```python
from build123d import *

# Parameters (mm, degrees)
SKETCH1_W                       = 150
SKETCH1_H                       = 40
BOSS_EXTRUDE1_DEPTH             = 2
SKETCH2_W                       = 150
SKETCH2_H                       = 40
BOSS_EXTRUDE2_DEPTH             = 2
CUT_EXTRUDE1_DEPTH              = 12.7
CUT_EXTRUDE1_DEPTH_BACK         = 2.3
BOSS_EXTRUDE3_DEPTH             = 9
BOSS_EXTRUDE4_REACH             = 32.803
BOSS_EXTRUDE4_DIRECTION_2_REACH = 11.197
CUT_EXTRUDE2_DEPTH              = 9
CUT_EXTRUDE3_DEPTH              = 2
SKETCH8_W                       = 10.5
SKETCH8_H                       = 9.597099162
SKETCH8_H_2                     = 6.297094949
BOSS_EXTRUDE5_DEPTH             = 9


with BuildPart() as part:
    # Sketch1 → Boss-Extrude1 (new body)
    with BuildSketch(Plane.XY):
        with Locations((53.542293618, 10.802935989)):
            Rectangle(SKETCH1_W, SKETCH1_H)
        with BuildLine():
            Line((107.411442145, 19.39470724), (107.411442145, 16.563139449))
            ThreePointArc((107.411442145, 16.563139449), (99.879507012, 8.827431039), (90.278173099, 3.889251358))
            ThreePointArc((90.278173099, 3.889251358), (87.976829975, 4.107947017), (85.862026946, 5.041550847))
            Line((85.862026946, 5.041550847), (83.564794922, 4.425052911))
            Line((83.564794922, 4.425052911), (81.157246557, 3.778949869))
            ThreePointArc((81.157246557, 3.778949869), (80.265596131, 1.871389792), (78.431111832, 0.8377103))
            Line((78.431111832, 0.8377103), (63.171073337, -3.257558326))
            ThreePointArc((63.171073337, -3.257558326), (60.782240037, -2.264409978), (59.531114294, 0))
            Line((59.531114294, 0), (51.260116039, 0))
            ThreePointArc((51.260116039, 0), (50.153419477, -2.317171365), (47.784117276, -3.307356952))
            Line((47.784117276, -3.307356952), (15.784117324, -3.309106743))
            ThreePointArc((15.784117324, -3.309106743), (13.343545232, -2.355539788), (12.195889194, 0))
            Line((12.195889194, 0), (0, 0))
            Line((0, 0), (0, 7.1))
            Line((0, 7.1), (11.639427583, 7.1))
            ThreePointArc((11.639427583, 7.1), (13.95708374, 11.772480363), (17.201849985, 15.85599537))
            ThreePointArc((17.201849985, 15.85599537), (17.97614749, 16.386455083), (18.8959739, 16.573119247))
            Line((18.8959739, 16.573119247), (44.695973562, 16.568946787))
            ThreePointArc((44.695973562, 16.568946787), (45.539742509, 16.358143902), (46.249834575, 15.85599537))
            ThreePointArc((46.249834575, 15.85599537), (49.049011998, 12.449181276), (51.19972816, 8.6))
            Line((51.19972816, 8.6), (59.697013712, 8.6))
            ThreePointArc((59.697013712, 8.6), (60.947722352, 11.657213146), (63.162897087, 14.107483583))
            ThreePointArc((63.162897087, 14.107483583), (63.865840812, 15.804539858), (65.562897087, 16.507483583))
            Line((65.562897087, 16.507483583), (72.962892379, 16.499136125))
            ThreePointArc((72.962892379, 16.499136125), (74.529247661, 15.732293003), (75.162897087, 14.107483583))
            ThreePointArc((75.162897087, 14.107483583), (76.943795958, 13.247586891), (78.431584017, 11.944701709))
            Line((78.431584017, 11.944701709), (84.544097467, 13.585089744))
            ThreePointArc((84.544097467, 13.585089744), (85.264438336, 15.182566708), (86.505516367, 16.419720272))
            ThreePointArc((86.505516367, 16.419720272), (94.138787289, 25.104262189), (104.023703334, 19.106218503))
            Line((104.023703334, 19.106218503), (107.411442145, 19.39470724))
        make_face(mode=Mode.SUBTRACT)
    extrude(amount=BOSS_EXTRUDE1_DEPTH)

    # Sketch2 → Boss-Extrude2 (add)
    with BuildSketch(Plane.XY):
        with Locations((53.542293618, 10.802935989)):
            Rectangle(SKETCH2_W, SKETCH2_H)
    extrude(amount=-BOSS_EXTRUDE2_DEPTH)

    # Sketch3 → Cut-Extrude1 (cut, two sides)
    with BuildSketch(Plane(origin=(0, 0, 0), x_dir=(1, 0, 0), z_dir=(0, 1, 0))) as cut_extrude1_sk:
        with BuildLine():
            Line((0, -0.8), (0, -17.6))
            ThreePointArc((0, -17.6), (-15.540418318, -9.2), (0, -0.8))
        make_face()
    extrude(amount=CUT_EXTRUDE1_DEPTH, mode=Mode.SUBTRACT)
    extrude(cut_extrude1_sk.sketch, amount=-CUT_EXTRUDE1_DEPTH_BACK, mode=Mode.SUBTRACT)

    # Sketch4 → Boss-Extrude3 (add)
    with BuildSketch(Plane.XY):
        Polygon((0, 7.1), (0, 12.7), (-12.497856815, 12.7), (-15.345436436, 12.7), (-15.345436436, 16.697099162), (-12.345546973, 16.697099162), (4, 16.697099162), (11, 16.697099162), (11, 7.1), align=None)
        Polygon((0, 0), (0, -2.3), (-12.497856815, -2.3), (-15.345436436, -2.3), (-15.345436436, -6.297094949), (-12.345436436, -6.297094949), (4, -6.297094949), (11, -6.297094949), (11, 0), align=None)
    extrude(amount=BOSS_EXTRUDE3_DEPTH)

    # Boss-Extrude4: up to this face of the body (flat: up to its plane)
    boss_extrude4_end = Plane(part.part.faces().sort_by_distance((-2.172718218, 16.697099162, 5.5))[0])
    # Sketch5 → Boss-Extrude4 (add, up to the picked face)
    with BuildSketch(Plane(origin=(0, 0, 0), x_dir=(1, 0, 0), z_dir=(0, 1, 0)), mode=Mode.PRIVATE) as boss_extrude4_sk1:
        with BuildLine():
            Line((-15.290812019, -9), (-19.400060853, -9))
            Line((-19.400060853, -9), (-19.400060853, -2))
            Line((-19.400060853, -2), (-12.345436436, -2))
            ThreePointArc((-12.345436436, -2), (-14.524477307, -5.20278927), (-15.290812019, -9))
        make_face()
    boss_extrude4_tool1 = split(extrude(boss_extrude4_sk1.sketch, amount=BOSS_EXTRUDE4_REACH, mode=Mode.PRIVATE), bisect_by=boss_extrude4_end, keep=Keep.BOTH, mode=Mode.PRIVATE)
    add(boss_extrude4_tool1.solids().sort_by_distance((-16.816054, 0, 5.171228))[0])

    # Boss-Extrude4 direction 2: up to this face of the body (flat: up to its plane)
    boss_extrude4_direction_2_end = Plane(part.part.faces().sort_by_distance((-2.172718218, -6.297094949, 5.5))[0])
    # Sketch5 → Boss-Extrude4 direction 2 (add, up to the picked face)
    with BuildSketch(Plane(origin=(0, 0, 0), x_dir=(1, 0, 0), z_dir=(0, 1, 0)), mode=Mode.PRIVATE) as boss_extrude4_direction_2_sk1:
        with BuildLine():
            Line((-15.290812019, -9), (-19.400060853, -9))
            Line((-19.400060853, -9), (-19.400060853, -2))
            Line((-19.400060853, -2), (-12.345436436, -2))
            ThreePointArc((-12.345436436, -2), (-14.524477307, -5.20278927), (-15.290812019, -9))
        make_face()
    boss_extrude4_direction_2_tool1 = split(extrude(boss_extrude4_direction_2_sk1.sketch, amount=-BOSS_EXTRUDE4_DIRECTION_2_REACH, mode=Mode.PRIVATE), bisect_by=boss_extrude4_direction_2_end, keep=Keep.BOTH, mode=Mode.PRIVATE)
    add(boss_extrude4_direction_2_tool1.solids().sort_by_distance((-16.816054, 0, 5.171228))[0])

    # Sketch6 → Cut-Extrude2 (cut)
    with BuildSketch(Plane.XY.offset(9)):
        Polygon((0, 7.1), (0, 12.7), (-15.290812019, 12.7), (-15.290812019, 13.2), (0.5, 13.2), (0.5, 7.1), align=None)
        Polygon((-15.290812019, -2.3), (0, -2.3), (0, 0), (0.5, 0), (0.5, -2.8), (-15.290812019, -2.8), align=None)
    extrude(amount=-CUT_EXTRUDE2_DEPTH, mode=Mode.SUBTRACT)

    # Sketch7 → Cut-Extrude3 (cut)
    with BuildSketch(Plane.XY.offset(2)):
        Polygon((11.639427583, 7.1), (11.639427583, 26.1), (109.411442143, 26.1), (109.411442143, -4.30823185), (11.639427583, -4.30823185), align=None)
    extrude(amount=-CUT_EXTRUDE3_DEPTH, mode=Mode.SUBTRACT)

    # Sketch8 → Boss-Extrude5 (add)
    with BuildSketch(Plane.XY.offset(9)):
        with Locations((5.75, 11.898549581)):
            Rectangle(SKETCH8_W, SKETCH8_H)
        with Locations((5.75, -3.148547475)):
            Rectangle(SKETCH8_W, SKETCH8_H_2)
    extrude(amount=BOSS_EXTRUDE5_DEPTH)


solid = part.part
```
Work out the finished part from the listing and answer in its coordinate system (mm). A direction names the side the tool comes from. Round coordinates to 2 decimals unless told otherwise and drop trailing zeros. Order: outer loops, then holes, each group sorted by start corner. A loop starts at its lowest first (then second) coordinate and runs counter-clockwise, first axis right, second up.
Q1. A cutting plane is placed at C-C, the plane x = 67.5. Determine the outline of the cut face in (y, z).
Solution:
outline: (-9.2, -2) - (30.8, -2) - (30.8, 2) - (26.1, 2) - (26.1, 0) - (-4.31, 0) - (-4.31, 2) - (-9.2, 2) - close
Q2. A cutting plane is placed at B-B, the plane y = 2.5. Determine the outline of the cut face in (x, z), then the cut area to 3 significant figures.
Solution:
outline: (-21.46, -2) - (128.54, -2) - (128.54, 2) - (109.41, 2) - (109.41, 0) - (0, 0) - (0, 0.8) arc R10.04 cw to (-12.5, 2) - (-12.35, 2) arc R9.79 cw to (-15.29, 9) - (-19.4, 9) - (-19.4, 2) - (-21.46, 2) - close
area: 390 mm2
Q3. Find the intervals of material crossed by line 1 along Y through (x, z) = (4, 7.5); line 2 along Y through (x, z) = (-6, 2.5); line 3 along Z through (x, y) = (91.5, 22), in increasing order.
Solution:
line 1: y = -6.3 to 0, 7.1 to 16.7
line 2: y = -6.3 to -2.8, 13.2 to 16.7
line 3: z = -2 to 0
Q4. Given pin 1 Ø3.5 at (x, z) = (8.5, 13.5) entering from +Y; pin 2 Ø5 at (x, y) = (17, 20) entering from +Z; pin 3 Ø9 at (x, z) = (5.5, 8.5) entering from -Y, each flat-ended and moving along its own axis, determine where each tip first touches the part or whether it passes through.
Solution:
pin 1: stops at y = 16.7
pin 2: stops at z = 0
pin 3: stops at y = -6.3
Q5. A cutting plane is placed at D-D, the plane z = 4. Determine the outline of the cut face in (x, y), then the cut area to 3 significant figures.
Solution:
outline: (-19.4, -6.3) - (11, -6.3) - (11, 0) - (0.5, 0) - (0.5, -2.8) - (-15.29, -2.8) - (-15.29, -2.3) - (-13.92, -2.3) - (-13.92, 12.7) - (-15.29, 12.7) - (-15.29, 13.2) - (0.5, 13.2) - (0.5, 7.1) - (11, 7.1) - (11, 16.7) - (-19.4, 16.7) - close
area: 392 mm2
Q6. A tool of negligible diameter and unlimited length cuts with its end or side. For faces 5 (the flat face through (52, -9.197, 0)), 6 (the flat face through (-1, -6.297, 8)), 7 (the flat face through (-7, -2.8, 5)), 8 (the flat face through (11, -3, 10)), from which of +Z, -Z, +X, -X, +Y, -Y can it reach the whole face along a straight path? Write none if from no direction.
Solution:
face 5: +Z, -Z, +X, -X, -Y
face 6: +Z, +X, -X, -Y
face 7: +Z
face 8: +Z, +X, +Y, -Y
Q7. A cutting plane is placed at A-A, the plane z = 10.75. Determine the outline of the cut face in (x, y).
Solution:
outline: (0.5, -6.3) - (11, -6.3) - (11, 0) - (0.5, 0) - close; (0.5, 7.1) - (11, 7.1) - (11, 16.7) - (0.5, 16.7) - close
Q8. The mould has two halves that part along Y. Classify faces 1 (the flat face through (-14, 12.7, 2)), 2 (the flat face through (-19.4, 5, 6)), 3 (the flat face through (0.5, -2, 11)), 4 (the flat face through (-1, 16.697, 8)): pulls with the +Y half, pulls with the -Y half, needs draft (parallel to the pull), parting line crosses it, or undercut.
Solution:
face 1: undercut
face 2: needs draft
face 3: undercut
face 4: pulls with the +Y half
